Here's how the part is built. I have some questions about the finished solid (model axes, mm). Coordinates: 2 decimals unless noted, no trailing zeros. Write each loop counter-clockwise with the first axis right and the second up, starting at its lowest first coordinate (ties: lowest second). Pieces come first, ordered by that corner, then holes. Notation, with made-up numbers: M -20,21.25 L 38,21.25 A23 cw 38,29.25 Z; hole C 14,1.25 d10. An arc over 180 degrees is marked long. Use a Markdown table: item, result.
```python
from build123d import *

# Parameters (mm, degrees)
PAD_DEPTH       = 2.7
SKETCH001_R     = 2.5
POCKET_DEPTH    = 5
SKETCH002_R     = 2.5
POCKET001_DEPTH = 5
SKETCH003_R     = 19.1
POCKET002_DEPTH = 5


with BuildPart() as part:
    # Sketch → Pad (new body)
    with BuildSketch(Plane.XY):
        with BuildLine():
            Line((40, 70.05), (40, 0))
            Line((40, 0), (-40, 0))
            Line((-40, 0), (-40, 70.05))
            ThreePointArc((40, 70.05), (0, 110.05), (-40, 70.05))
        make_face()
    extrude(amount=PAD_DEPTH)

    # Sketch001 → Pocket (cut)
    with BuildSketch(Plane.XY.offset(2.7)):
        with Locations((33.333, 70.05)):
            Circle(SKETCH001_R)
        with Locations((23, 22.5)):
            Circle(SKETCH001_R)
    pocket = extrude(amount=-POCKET_DEPTH, mode=Mode.SUBTRACT)

    # Mirrored: Pocket across Sketch001 V_Axis
    add(pocket.mirror(Plane(origin=(0, 0, 2.7), x_dir=(0, 0, 1), z_dir=(1, 0, 0))), mode=Mode.SUBTRACT)

    # Sketch002 → Pocket001 (cut)
    with BuildSketch(Plane.XY.offset(2.7)):
        with Locations((0, 103.4)):
            Circle(SKETCH002_R)
    extrude(amount=-POCKET001_DEPTH, mode=Mode.SUBTRACT)

    # Sketch003 → Pocket002 (cut)
    with BuildSketch(Plane.XY.offset(2.7)):
        with Locations((0, 70.05)):
            Circle(SKETCH003_R)
    extrude(amount=-POCKET002_DEPTH, mode=Mode.SUBTRACT)


solid = part.part
```
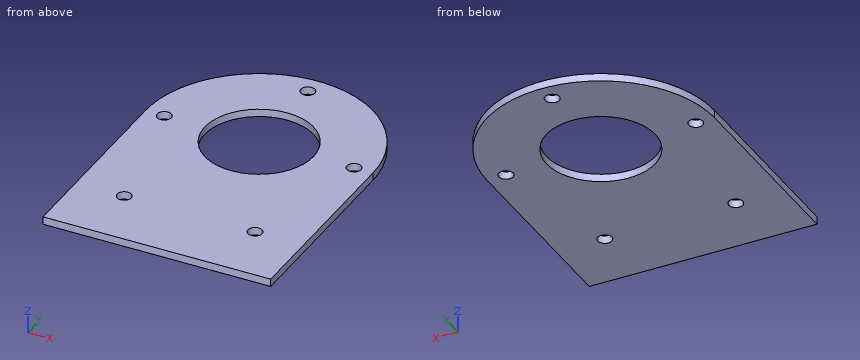
1. Suppose I cut it at C-C on x = -23. Write out the boundary of the cut face in (y, z).
Answers follow:
| item | result |
|---|---|
| outline | M 0,0 L 20,0 L 20,2.7 L 0,2.7 Z; M 25,0 L 102.78,0 L 102.78,2.7 L 25,2.7 Z |
2. I need wall thicknesses on probe 1 along Y at (x, z) = (0, 1.15); probe 2 along X at (y, z) = (72, 2.4); probe 3 along Y at (x, z) = (-23, 1.3). Which ranges of each line are inside material? Lowest first, please.
Answers follow:
| item | result |
|---|---|
| probe 1 | y = 0 to 50.95, 89.15 to 100.9, 105.9 to 110.05 |
| probe 2 | x = -39.95 to -34.9, -31.77 to -19, 19 to 31.77, 34.9 to 39.95 |
| probe 3 | y = 0 to 20, 25 to 102.78 |
3. Suppose I cut it at B-B on z = 1.3. Write out the boundary of the cut face in (x, y), and give its area (3 significant figures).
Answers follow:
| item | result |
|---|---|
| outline | M -40,0 L 40,0 L 40,70.05 A40 ccw -40,70.05 Z; hole C -33.33,70.05 d5; hole C -23,22.5 d5; hole C 0,70.05 d38.2; hole C 0,103.4 d5; hole C 23,22.5 d5; hole C 33.33,70.05 d5 |
| area | 6,870 mm2 |
4. Suppose I cut it at A-A on y = 22.5. Write out the boundary of the cut face in (x, z).
Answers follow:
| item | result |
|---|---|
| outline | M -40,0 L -25.5,0 L -25.5,2.7 L -40,2.7 Z; M -20.5,0 L 20.5,0 L 20.5,2.7 L -20.5,2.7 Z; M 25.5,0 L 40,0 L 40,2.7 L 25.5,2.7 Z |
5. Will these pins go through, and if not, where does the flat tip stop? pin 1 Ø3 at (x, y) = (-33.333, 70.05) entering from -Z; pin 2 Ø1.5 at (x, z) = (23, 1.5) entering from +Y.
Answers follow:
| item | result |
|---|---|
| pin 1 | passes through |
| pin 2 | stops at y = 103.29 |
6. Suppose I cut it at D-D on y = 61.5. Write out the boundary of the cut face in (x, z), and give its area (3 significant figures).
Answers follow:
| item | result |
|---|---|
| outline | M -40,0 L -17.08,0 L -17.08,2.7 L -40,2.7 Z; M 17.08,0 L 40,0 L 40,2.7 L 17.08,2.7 Z |
| area | 124 mm2 |
